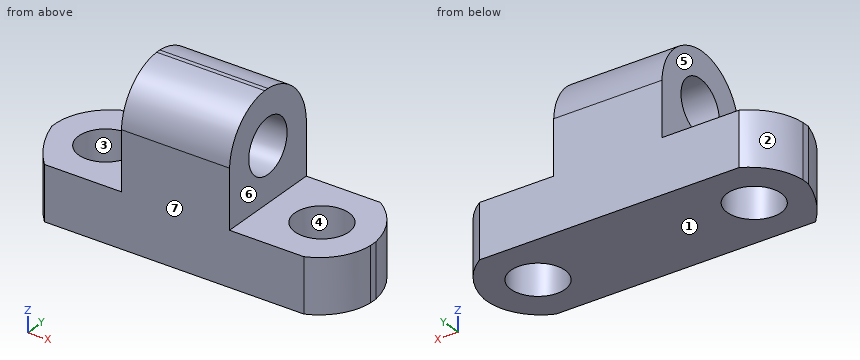
from build123d import *

# Parameters (mm, degrees)
F1_DEPTH  = 25.4
F2_R      = 6.35
F3_DEPTH  = 25.4
F4_R      = 6.35
F5_DEPTH  = 25.4
F6_R      = 6.35
F7_DEPTH  = 25.4
F9_DEPTH  = 25.4
F11_DEPTH = 25.4
F13_DEPTH = 25.4


with BuildPart() as f1:
    # F0 (on Front) → F1 (new body)
    with BuildSketch(Plane.XZ):
        Polygon((0, 12.7), (0, 0), (76.2, 0), (76.2, 12.7), (50.8, 12.7), (50.8, 38.1), (25.4, 38.1), (25.4, 12.7), align=None)
    extrude(amount=F1_DEPTH)

    # F2 (on face) → F3 (cut)
    with BuildSketch(Plane.XY.offset(12.7)):
        with Locations((63.5, -12.7)):
            Circle(F2_R)
    extrude(amount=-F3_DEPTH, mode=Mode.SUBTRACT)

    # F4 (on face) → F5 (cut)
    with BuildSketch(Plane.XY.offset(12.7)):
        with Locations((12.7, -12.7)):
            Circle(F4_R)
    extrude(amount=-F5_DEPTH, mode=Mode.SUBTRACT)

    # F6 (on face) → F7 (cut)
    with BuildSketch(Plane.YZ.offset(50.8)):
        with Locations((-12.7, 25.4)):
            Circle(F6_R)
    extrude(amount=-F7_DEPTH, mode=Mode.SUBTRACT)

    # F8 (on face) → F9 (cut)
    with BuildSketch(Plane.XY.offset(12.7)):
        with BuildLine():
            ThreePointArc((68.2354718447, 0), (73.6121400289, -5.4755298609), (76.2, -12.7))
            Line((76.2, -12.7), (76.2, 0))
            Line((76.2, 0), (68.2354718447, 0))
        make_face()
        with BuildLine():
            ThreePointArc((76.2, -14.5233565668), (73.7819264131, -21.1070720145), (68.2354718447, -25.4))
            Line((68.2354718447, -25.4), (76.2, -25.4))
            Line((76.2, -25.4), (76.2, -14.5233565668))
        make_face()
    extrude(amount=-F9_DEPTH, mode=Mode.SUBTRACT)

    # F10 (on face) → F11 (cut)
    with BuildSketch(Plane.XY.offset(12.7)):
        with BuildLine():
            ThreePointArc((0, -10.8889817229), (2.2004439823, -4.4673896083), (7.3113371618, 0))
            Line((7.3113371618, 0), (0, 0))
            Line((0, 0), (0, -10.8889817229))
        make_face()
        with BuildLine():
            ThreePointArc((7.3113371618, -25.4), (2.9064077234, -19.4813463584), (0, -12.7))
            Line((0, -12.7), (0, -25.4))
            Line((0, -25.4), (7.3113371618, -25.4))
        make_face()
    extrude(amount=-F11_DEPTH, mode=Mode.SUBTRACT)

    # F12 (on face) → F13 (cut)
    with BuildSketch(Plane.YZ.offset(50.8)):
        with BuildLine():
            Line((0, 38.1), (-12.7, 38.1))
            ThreePointArc((-12.7, 38.1), (-3.9193677073, 34.1806322927), (0, 25.4))
            Line((0, 25.4), (0, 38.1))
        make_face()
        with BuildLine():
            ThreePointArc((-25.4, 26.4494707513), (-21.8419395594, 34.5419395594), (-13.7494707513, 38.1))
            Line((-13.7494707513, 38.1), (-25.4, 38.1))
            Line((-25.4, 38.1), (-25.4, 26.4494707513))
        make_face()
    extrude(amount=-F13_DEPTH, mode=Mode.SUBTRACT)


solid = f1.part
Could you check a few things on this model? Use its own coordinates, in mm. Face numbers are marked on the shaded views. A direction names the side the tool comes from. Round coordinates to 2 decimals unless told otherwise and drop trailing zeros. Loops run counter-clockwise (first coordinate to the right, second up) from the corner with the lowest first, then second, coordinate; pieces in that order, holes last. Notation, with made-up numbers: (26.25, 40.5) - (61.25, 40.5) arc R21 ccw to (61.25, 64.5) - close; hole circle Ø6 at (75.25, 52). An arc over 180 degrees is marked (long way). Write item = value, one per line.
1) If we mould it in two halves opening along X, with no side actions, what happens to the marked faces 1, 2, 3 and 4? For each: pulls with the +X half, pulls with the -X half, needs draft (parallel to the pull), parting line crosses it, or undercut.
Computed:
face_1 = needs draft
face_2 = pulls with the -X half
face_3 = undercut
face_4 = undercut
2) Imagine slicing it at C-C (y = -8.5). Please give me the cut outline in (x, z), and give its area (3 significant figures).
Computed:
outline = (0.39, 0) - (7.94, 0) - (7.94, 12.7) - (0.39, 12.7) - close; (17.46, 0) - (58.74, 0) - (58.74, 12.7) - (50.8, 12.7) - (50.8, 20.64) - (25.4, 20.64) - (25.4, 12.7) - (17.46, 12.7) - close; (25.4, 30.16) - (50.8, 30.16) - (50.8, 37.18) - (25.4, 37.18) - close; (68.26, 0) - (75.13, 0) - (75.13, 12.7) - (68.26, 12.7) - close
area = 1,090 mm2
3) I need wall thicknesses on line 1 along Y through (x, z) = (39, 25); line 2 along Y through (x, z) = (34.5, 22.5); line 3 along Z through (x, y) = (42.5, -12.7). Which ranges of each line are inside material? Lowest first, please. Write a range as from..to.
Computed:
line_1 = -25.4..-19.04, -6.36..0
line_2 = -25.4..-18.35, -7.05..0
line_3 = 0..19.05, 31.75..38.1
4) I'm going to push flat-ended pins straight in: P1, Ø14.5, axis at x = 12.7, y = -12.7, coming from the +Z side; P2, Ø8, axis at y = -13.5, z = 20, coming from the +X side; P3, Ø6, axis at y = -22, z = 9, coming from the -X side. Where does each tip first touch, or does it pass through?
Computed:
P1 = 12.7
P2 = 50.8
P3 = 2.63
5) On a 3-axis mill with a long thin cutter (end or side, diameter ignored), from which of +Z, -Z, +X, -X, +Y, -Y can I reach the whole of each face in a straight line? I mean the marked faces 5, 6 and 7. Say none if no direction works.
Computed:
face_5 = +Z, -X, +Y, -Y
face_6 = +Z, +X, +Y, -Y
face_7 = +Z, -Z, +X, -X, -Y
6) Imagine slicing it at D-D (x = 37.5). Please give me the cut outline in (y, z), and give its area (3 significant figures).
Computed:
outline = (-25.4, 0) - (0, 0) - (0, 25.4) arc R13.45 ccw to (-12.7, 38.1) - (-13.75, 38.1) arc R12.19 ccw to (-25.4, 26.45) - close; hole circle Ø12.7 at (-12.7, 25.4)
area = 771 mm2
7) Imagine slicing it at B-B (z = 10.5). Please give me the cut outline in (x, y), and give its area (3 significant figures).
Computed:
outline = (0, -12.7) arc R31.48 ccw to (7.31, -25.4) - (68.24, -25.4) arc R12.69 ccw to (76.2, -14.52) - (76.2, -12.7) arc R17.89 ccw to (68.24, 0) - (7.31, 0) arc R13.14 ccw to (0, -10.89) - close; hole circle Ø12.7 at (12.7, -12.7); hole circle Ø12.7 at (63.5, -12.7)
area = 1,560 mm2
8) Imagine slicing it at A-A (x = 63.5). Please give me the cut outline in (y, z).
Computed:
outline = (-25.4, 0) - (-19.05, 0) - (-19.05, 12.7) - (-25.4, 12.7) - close; (-6.35, 0) - (0, 0) - (0, 12.7) - (-6.35, 12.7) - close
